The model under review builds one solid part; all positions refer to its coordinate system, in mm. Face numbers are marked on the shaded views. A direction names the side the tool comes from. Give positions to 0.01 mm unless a question says otherwise; leave off trailing zeros. Write each loop counter-clockwise with the first axis right and the second up, starting at its lowest first coordinate (ties: lowest second). Pieces come first, ordered by that corner, then holes. Notation, with made-up numbers: M 20,32 L 70,32 A23 cw 70,59 Z; hole C -37,-2.75 d10. An arc over 180 degrees is marked long. Write each question's results on one line, items separated by ' | '. Start each with the question number.
from build123d import *

# Parameters (mm, degrees)
F0_R     = 12.7
F1_DEPTH = 25
F2_R     = 10.5
F3_DEPTH = 6
F4_SIZE  = 1
F6_D     = 8
F6_DEPTH = 18
F6_TIP   = 2.4034424761


with BuildPart() as f1:
    # F0 (on Front) → F1 (new body)
    with BuildSketch(Plane.XZ):
        Circle(F0_R)
    extrude(amount=F1_DEPTH)

    # F2 (on face) → F3 (join)
    with BuildSketch(Plane.XZ.offset(25)):
        Circle(F2_R)
    extrude(amount=F3_DEPTH)

    # F4
    f4_edges = [f1.edges().sort_by_distance(p)[0] for p in [
        (-10.5, -31, 0),
        (-12.7, 0, 0),
    ]]
    chamfer(f4_edges, length=F4_SIZE)

    # F6
    with Locations(Plane(origin=(0, 0, 0), x_dir=(-1, 0, 0), z_dir=(0, 1, 0))):
        with Locations((0, 0)):
            Hole(F6_D / 2, depth=F6_DEPTH)
            with Locations((0, 0, -(F6_DEPTH + F6_TIP / 2))):  # 118° drill point
                Cone(0, F6_D / 2, F6_TIP, mode=Mode.SUBTRACT)


solid = f1.part
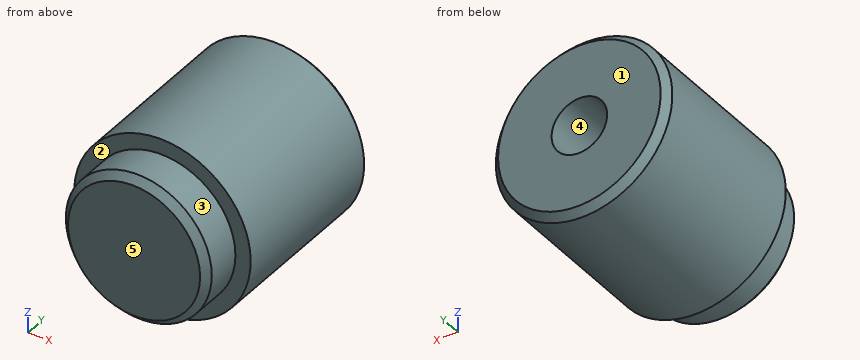
(1) Draft analysis for pull direction X (two halves, no side actions). For the marked faces 3, 4 and 5, state which applies: pulls with the +X half, pulls with the -X half, needs draft (parallel to the pull), parting line crosses it, or undercut.
(2) Clearance check with flat-ended pins moving along their axes: P1, Ø4, axis at x = 3, y = -12, coming from the +Z side; P2, Ø8, axis at x = 4.5, y = -11.5, coming from the -Z side; P3, Ø8, axis at y = -21, z = -6.5, coming from the -X side. State where each tip first meets the part, or that it passes through.
(3) Add section B-B (y = -29). State the section outline as (x, z) points, then the cut area to 3 significant figures.
(4) Add section A-A (y = -9.5). State the section outline as (x, z) points.
(5) Wall thickness on L1, parallel to Z at x = 0, y = -13.75; L2, parallel to Z at x = 1.5, y = -4.5; L3, parallel to Y at x = -3, z = -11: over which ranges is each line inside the solid? List them lowest first.
(6) Machinability: for the marked faces 1 and 2, which of the approach directions +Z, -Z, +X, -X, +Y, -Y give a long, thin tool a straight path to every point of the face, cutting with its end or side? Answer none if there is none.
Calculated:
1) face 3: parting line crosses it | face 4: undercut | face 5: needs draft
2) P1: stops at z = 12.66 | P2: stops at z = -12.69 | P3: stops at x = -12.45
3) outline: C 0,0 d21 | area: 346 mm²
4) outline: C 0,0 d25.4; hole C 0,0 d8
5) L1: z = -12.7 to -4, 4 to 12.7 | L2: z = -12.61 to -3.71, 3.71 to 12.61 | L3: y = -25 to 0
6) face 1: +Z, -Z, +X, -X, +Y | face 2: -Y
